Source: CAD feature listing. Evaluate the final solid. Frame: model axes, mm. Face numbers are marked on the shaded views. A direction names the side the tool comes from. Give positions to 0.01 mm unless a question says otherwise; leave off trailing zeros. Write each loop counter-clockwise with the first axis right and the second up, starting at its lowest first coordinate (ties: lowest second). Pieces come first, ordered by that corner, then holes. Notation, with made-up numbers: (57.25, 75.25) - (97.25, 75.25) arc R32 ccw to (97.25, 108.25) - close; hole circle Ø4 at (-12, 61). An arc over 180 degrees is marked (long way). Answer as a JSON object with one key per item and string values. Group by question number.
from build123d import *

# Parameters (mm, degrees)
SKETCH1_R           = 20
BOSS_EXTRUDE1_DEPTH = 5
SKETCH2_R           = 10
BOSS_EXTRUDE2_DEPTH = 5
SKETCH3_R           = 20
BOSS_EXTRUDE3_DEPTH = 5
SKETCH4_R           = 3
CUT_EXTRUDE1_DEPTH  = 33.015621187


with BuildPart() as part:
    # Sketch1 → Boss-Extrude1 (new body)
    with BuildSketch(Plane.XY):
        Circle(SKETCH1_R)
    extrude(amount=BOSS_EXTRUDE1_DEPTH)

    # Sketch2 → Boss-Extrude2 (add)
    with BuildSketch(Plane.XY.offset(5)):
        Circle(SKETCH2_R)
    extrude(amount=BOSS_EXTRUDE2_DEPTH)

    # Sketch3 → Boss-Extrude3 (add)
    with BuildSketch(Plane.XY.offset(10)):
        Circle(SKETCH3_R)
    extrude(amount=BOSS_EXTRUDE3_DEPTH)

    # Sketch4 → Cut-Extrude1 (cut, through all)
    with BuildSketch(Plane.XY.offset(15)):
        Circle(SKETCH4_R)
    extrude(amount=-CUT_EXTRUDE1_DEPTH, mode=Mode.SUBTRACT)


solid = part.part
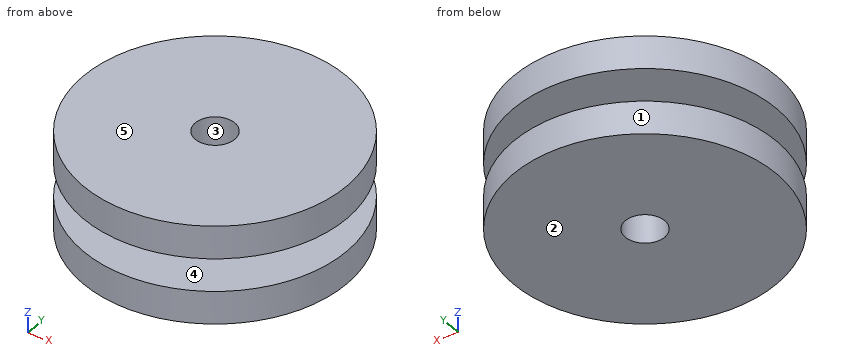
Q1. Section C-C on z = 5.5. Return the cut outline in (x, y).
Q2. Draft query along X for the marked faces 1, 2 and 3. Return one class per face: released by +X, released by -X, zero draft, split by the parting line, or undercut.
Q3. First-contact query: pin 1 Ø1 at (y, z) = (13, 3) entering from +X; pin 2 Ø6 at (y, z) = (13.5, 11) entering from -X; pin 3 Ø5 at (y, z) = (5, 11.5) entering from +X. Flat tips, straight axial feed; report the tip coordinate or a pass-through.
Q4. Reachability of the marked faces 4 and 5 from +Z, -Z, +X, -X, +Y, -Y: full face, straight path, thin tool, end or side. Return the list, or none.
Q5. Section A-A on x = 0. Return the cut outline in (y, z), then the cut area to 3 significant figures.
Q6. Ray query, probe 1 along Y at (x, z) = (0, 8.5); probe 2 along Y at (x, z) = (0, 11.5); probe 3 along Z at (x, y) = (-14, 14). Return the intervals inside material, ascending. Write a range as [from, to].
Q7. Section D-D on y = -5.5. Return the cut outline in (x, z), then the cut area to 3 significant figures.
Taken from the geometry:
{
 "1": {"outline": "circle Ø20 at (0, 0); hole circle Ø6 at (0, 0)"},
 "2": {"face 1": "split by the parting line", "face 2": "zero draft", "face 3": "undercut"},
 "3": {"pin 1": "stops at x = 15.61", "pin 2": "stops at x = -17.02", "pin 3": "stops at x = 19.84"},
 "4": {"face 4": "none", "face 5": "+Z, +X, -X, +Y, -Y"},
 "5": {"outline": "(-20, 0) - (-3, 0) - (-3, 15) - (-20, 15) - (-20, 10) - (-10, 10) - (-10, 5) - (-20, 5) - close; (3, 0) - (20, 0) - (20, 5) - (10, 5) - (10, 10) - (20, 10) - (20, 15) - (3, 15) - close", "area": "410 mm²"},
 "6": {"probe 1": "y = [-10, -3], [3, 10]", "probe 2": "y = [-20, -3], [3, 20]", "probe 3": "z = [0, 5], [10, 15]"},
 "7": {"outline": "(-19.23, 0) - (19.23, 0) - (19.23, 5) - (8.35, 5) - (8.35, 10) - (19.23, 10) - (19.23, 15) - (-19.23, 15) - (-19.23, 10) - (-8.35, 10) - (-8.35, 5) - (-19.23, 5) - close", "area": "468 mm²"}
}
